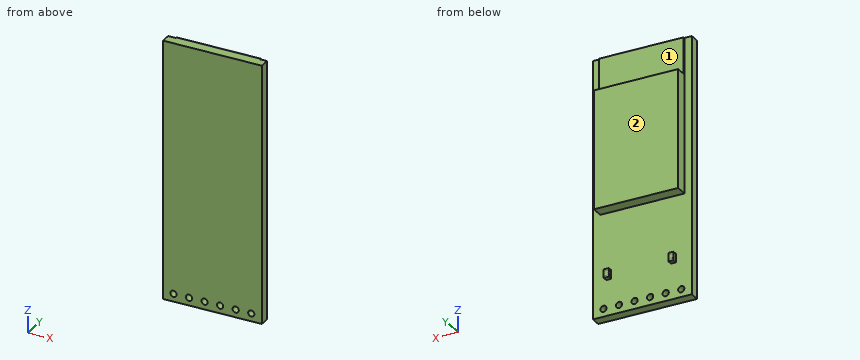
from build123d import *

# Parameters (mm, degrees)
SKETCH1_W           = 16.1544
SKETCH1_H           = 42.037
BOSS_EXTRUDE1_DEPTH = 0.8001
SKETCH2_R           = 0.508
CUT_EXTRUDE1_DEPTH  = 1.6002
SKETCH3_W           = 13.75
SKETCH3_H           = 25.275
BOSS_EXTRUDE2_DEPTH = 0.3
SKETCH4_W           = 13.75
SKETCH4_H           = 19.35
BOSS_EXTRUDE3_DEPTH = 1.625
SKETCH5_W           = 0.82
SKETCH5_H           = 1.4
BOSS_EXTRUDE4_DEPTH = 0.75
SKETCH6_R           = 0.41
BOSS_EXTRUDE5_DEPTH = 0.01


with BuildPart() as part:
    # Sketch1 → Boss-Extrude1 (new body, symmetric)
    with BuildSketch(Plane(origin=(0, 0, 0), x_dir=(1, 0, 0), z_dir=(0, 1, 0))):
        Rectangle(SKETCH1_W, SKETCH1_H)
    extrude(amount=BOSS_EXTRUDE1_DEPTH, both=True)

    # Sketch2 → Cut-Extrude1 (cut)
    with BuildSketch(Plane(origin=(0, 0.8001, 0), x_dir=(1, 0, 0), z_dir=(0, 1, 0))):
        with Locations((-6.35, 19.7485)):
            Circle(SKETCH2_R)
        with Locations((-3.81, 19.7485)):
            Circle(SKETCH2_R)
        with Locations((-1.27, 19.7485)):
            Circle(SKETCH2_R)
        with Locations((1.27, 19.7485)):
            Circle(SKETCH2_R)
        with Locations((3.81, 19.7485)):
            Circle(SKETCH2_R)
        with Locations((6.35, 19.7485)):
            Circle(SKETCH2_R)
    extrude(amount=-CUT_EXTRUDE1_DEPTH, mode=Mode.SUBTRACT)

    # Sketch3 → Boss-Extrude2 (add)
    with BuildSketch(Plane(origin=(0, 0.8001, 0), x_dir=(1, 0, 0), z_dir=(0, 1, 0))):
        with Locations((0, -8.331)):
            Rectangle(SKETCH3_W, SKETCH3_H)
    extrude(amount=BOSS_EXTRUDE2_DEPTH)

    # Sketch4 → Boss-Extrude3 (add)
    with BuildSketch(Plane(origin=(0, 1.1001, 0), x_dir=(1, 0, 0), z_dir=(0, 1, 0))):
        with Locations((0, -5.3685)):
            Rectangle(SKETCH4_W, SKETCH4_H)
    extrude(amount=BOSS_EXTRUDE3_DEPTH)

    # Sketch5 → Boss-Extrude4 (add)
    with BuildSketch(Plane(origin=(0, 0.8001, 0), x_dir=(1, 0, 0), z_dir=(0, 1, 0))):
        with Locations((-5.0672, 14.4685)):
            Rectangle(SKETCH5_W, SKETCH5_H)
        with Locations((5.4872, 14.4685)):
            Rectangle(SKETCH5_W, SKETCH5_H)
    extrude(amount=BOSS_EXTRUDE4_DEPTH)

    # Sketch6 → Boss-Extrude5 (add)
    with BuildSketch(Plane(origin=(0, 1.5501, 0), x_dir=(1, 0, 0), z_dir=(0, 1, 0))):
        with Locations((-5.0672, 14.4685)):
            Circle(SKETCH6_R)
        with Locations((5.4872, 14.4685)):
            Circle(SKETCH6_R)
    extrude(amount=BOSS_EXTRUDE5_DEPTH)


solid = part.part
Geometry check sheet. Reference: the model listing, model coordinates, mm. Face numbers are marked on the shaded views. A direction names the side the tool comes from. Coordinates: 2 decimals unless noted, no trailing zeros. Order: outer loops, then holes, each group sorted by start corner. A loop starts at its lowest first (then second) coordinate and runs counter-clockwise, first axis right, second up. Notation, with made-up numbers: (-15, 36.25) -> (4, 36.25) arc R14 cw to (4, 42.25) -> close; hole circle Ø6 at (29.5, -28). An arc over 180 degrees is marked (long way). Use a Markdown table: item, result. Add a question column.
1. Cross-section at A-A (x = -1.27). Enter the section's corners in (y, z).
2. Material ranges on L1, parallel to Z at x = -1.27, y = -0.25; L2, parallel to Y at x = 3.5, z = -14; L3, parallel to X at y = 1.5, z = 1.5 (3 decimals), recorded low to high.
3. Cross-section at B-B (z = 5). Enter the section's corners in (x, y) (3 decimals), and give its area (3 significant figures).
4. Set-up check for the marked faces 1 and 2: record each of +Z, -Z, +X, -X, +Y, -Y from which the full face is reachable in a straight line by a thin tool's end or side.
5. Cross-section at C-C (y = 2.2). Enter the section's corners in (x, z) (1 decimal).
6. Cross-section at D-D (z = -10). Enter the section's corners in (x, y).
7. Go/stop test with flat-tipped pins: pin 1 Ø1.5 at (x, y) = (-1, 2) entering from -Z; pin 2 Ø0.6 at (x, z) = (-5, -14.5) entering from +Y; pin 3 Ø2 at (y, z) = (2, 12) entering from +X (3 decimals). Record where each tip stops, or that it passes through.
Filled sheet:
| question | item | result |
|---|---|---|
| 1 | outline | (-0.8, -21.02) -> (0.8, -21.02) -> (0.8, -20.26) -> (-0.8, -20.26) -> close; (-0.8, -19.24) -> (0.8, -19.24) -> (0.8, -4.31) -> (2.73, -4.31) -> (2.73, 15.04) -> (1.1, 15.04) -> (1.1, 20.97) -> (0.8, 20.97) -> (0.8, 21.02) -> (-0.8, 21.02) -> close |
| 2 | L1 | -21.02 to -20.26, -19.24 to 21.02 |
| 2 | L2 | -0.8 to 0.8 |
| 2 | L3 | -6.875 to 6.875 |
| 3 | outline | (-8.077, -0.8) -> (8.077, -0.8) -> (8.077, 0.8) -> (6.875, 0.8) -> (6.875, 2.725) -> (-6.875, 2.725) -> (-6.875, 0.8) -> (-8.077, 0.8) -> close |
| 3 | area | 52.3 mm2 |
| 4 | face 1 | +Z, +X, -X, +Y |
| 4 | face 2 | +Z, -Z, +X, -X, +Y |
| 5 | outline | (-6.9, -4.3) -> (6.9, -4.3) -> (6.9, 15) -> (-6.9, 15) -> close |
| 6 | outline | (-8.08, -0.8) -> (8.08, -0.8) -> (8.08, 0.8) -> (-8.08, 0.8) -> close |
| 7 | pin 1 | z = -4.31 |
| 7 | pin 2 | y = 1.56 |
| 7 | pin 3 | x = 6.875 |
